from build123d import *

# Parameters (mm, degrees)
SKETCH1_W           = 55
SKETCH1_H           = 50
SKETCH1_R           = 6
SKETCH1_R_2         = 1.5
BOSS_EXTRUDE1_DEPTH = 5
SKETCH2_W           = 5.5
SKETCH2_H           = 2
SKETCH2_W_2         = 3
SKETCH2_H_2         = 12
CUT_EXTRUDE1_DEPTH  = 5
SKETCH3_W           = 5
SKETCH3_H           = 60
SKETCH3_W_2         = 26.5
SKETCH3_H_2         = 5
BOSS_EXTRUDE2_DEPTH = 5


with BuildPart() as part:
    # Sketch1 → Boss-Extrude1 (new body)
    with BuildSketch(Plane.XY):
        with Locations((0, -2)):
            Rectangle(SKETCH1_W, SKETCH1_H)
        with Locations((0, -7)):
            Circle(SKETCH1_R, mode=Mode.SUBTRACT)
        with Locations((-15.5, 0)):
            Circle(SKETCH1_R_2, mode=Mode.SUBTRACT)
        with Locations((-7.75, 13.423393759)):
            Circle(SKETCH1_R_2, mode=Mode.SUBTRACT)
        with Locations((7.75, 13.423393759)):
            Circle(SKETCH1_R_2, mode=Mode.SUBTRACT)
        with Locations((15.5, 0)):
            Circle(SKETCH1_R_2, mode=Mode.SUBTRACT)
        with Locations((7.75, -13.423393759)):
            Circle(SKETCH1_R_2, mode=Mode.SUBTRACT)
        with Locations((-7.75, -13.423393759)):
            Circle(SKETCH1_R_2, mode=Mode.SUBTRACT)
    extrude(amount=BOSS_EXTRUDE1_DEPTH)

    # Sketch2 → Cut-Extrude1 (cut)
    with BuildSketch(Plane.XY.offset(5)):
        with Locations((-19.75, -21)):
            Rectangle(SKETCH2_W, SKETCH2_H)
        with Locations((19.75, -21)):
            Rectangle(SKETCH2_W, SKETCH2_H)
        with Locations((-19.75, -21)):
            Rectangle(SKETCH2_W_2, SKETCH2_H_2)
        with Locations((19.75, -21)):
            Rectangle(SKETCH2_W_2, SKETCH2_H_2)
        with Locations((19.75, 17)):
            Rectangle(SKETCH2_W_2, SKETCH2_H_2)
        with Locations((-19.75, 17)):
            Rectangle(SKETCH2_W_2, SKETCH2_H_2)
        with Locations((19.75, 17)):
            Rectangle(SKETCH2_W, SKETCH2_H)
        with Locations((-19.75, 17)):
            Rectangle(SKETCH2_W, SKETCH2_H)
    extrude(amount=-CUT_EXTRUDE1_DEPTH, mode=Mode.SUBTRACT)

    # Sketch3 → Boss-Extrude2 (add)
    with BuildSketch(Plane.XY.offset(5)):
        with Locations((-28.75, -2)):
            Rectangle(SKETCH3_W, SKETCH3_H)
        with Locations((0, -29.5)):
            Rectangle(SKETCH3_W_2, SKETCH3_H_2)
        with Locations((28.75, -2)):
            Rectangle(SKETCH3_W, SKETCH3_H)
        with Locations((0, 25.5)):
            Rectangle(SKETCH3_W_2, SKETCH3_H_2)
    extrude(amount=-BOSS_EXTRUDE2_DEPTH)


solid = part.part
Input: part model. Units: mm. Frame: model coordinates. A direction names the side the tool comes from. Round coordinates to 2 decimals unless told otherwise and drop trailing zeros. Order: outer loops, then holes, each group sorted by start corner. A loop starts at its lowest first (then second) coordinate and runs counter-clockwise, first axis right, second up. Notation, with made-up numbers: (35, 74) - (53, 74) arc R30 ccw to (53, 113) - close; hole circle Ø6 at (27.5, 56.5). An arc over 180 degrees is marked (long way). Use a Markdown table: item, result.
1. Section D-D on y = 19. Return the cut outline in (x, z).
Evaluation:
| item | result |
|---|---|
| outline | (-31.25, 0) - (-21.25, 0) - (-21.25, 5) - (-31.25, 5) - close; (-18.25, 0) - (18.25, 0) - (18.25, 5) - (-18.25, 5) - close; (21.25, 0) - (31.25, 0) - (31.25, 5) - (21.25, 5) - close |
2. Material intervals for probe 1 along X at (y, z) = (-25, 3.65); probe 2 along Y at (x, z) = (7.75, 1.95); probe 3 along X at (y, z) = (-27.5, 1.35), sorted ascending.
Evaluation:
| item | result |
|---|---|
| probe 1 | -31.25 to -21.25, -18.25 to 18.25, 21.25 to 31.25 |
| probe 2 | -32 to -14.92, -11.92 to 11.92, 14.92 to 28 |
| probe 3 | -31.25 to -26.25, -13.25 to 13.25, 26.25 to 31.25 |
3. Section C-C on x = -7.75. Return the cut outline in (y, z).
Evaluation:
| item | result |
|---|---|
| outline | (-32, 0) - (-14.92, 0) - (-14.92, 5) - (-32, 5) - close; (-11.92, 0) - (11.92, 0) - (11.92, 5) - (-11.92, 5) - close; (14.92, 0) - (28, 0) - (28, 5) - (14.92, 5) - close |
4. Access query for faces 4 (the face through (21.25, 20, 3)), 5 (the face through (22.5, -21, 3)), 6 (the face through (-31.25, -2, 3)), 7 (the face through (-16, -27, 2)), 8 (the face through (31.25, -2, 3)). Directions: +Z, -Z, +X, -X, +Y, -Y. A direction counts if a zero-diameter tool reaches every point of the face in a straight line with its end or side. Return the directions, or none.
Evaluation:
| item | result |
|---|---|
| face 4 | +Z, -Z, +Y |
| face 5 | +Z, -Z |
| face 6 | +Z, -Z, -X, +Y, -Y |
| face 7 | +Z, -Z, -Y |
| face 8 | +Z, -Z, +X, +Y, -Y |
5. Section A-A on x = -15.5. Return the cut outline in (y, z), then the cut area to 3 significant figures.
Evaluation:
| item | result |
|---|---|
| outline | (-27, 0) - (-1.5, 0) - (-1.5, 5) - (-27, 5) - close; (1.5, 0) - (23, 0) - (23, 5) - (1.5, 5) - close |
| area | 235 mm^2 |
6. Section B-B on y = -7. Return the cut outline in (x, z), then the cut area to 4 significant figures.
Evaluation:
| item | result |
|---|---|
| outline | (-31.25, 0) - (-6, 0) - (-6, 5) - (-31.25, 5) - close; (6, 0) - (31.25, 0) - (31.25, 5) - (6, 5) - close |
| area | 252.5 mm^2 |
7. First-contact query: pin 1 (1 mm diameter, centred on x = 17.5, z = 3, fed in from +Y); pin 2 (2.5 mm diameter, centred on x = 23, z = 2, fed in from -Y). Flat tips, straight axial feed; report the tip coordinate or a pass-through.
Evaluation:
| item | result |
|---|---|
| pin 1 | y = 23 |
| pin 2 | y = -27 |
8. Mould query, pull axis Y, two halves, no side actions, for faces 1 (the face through (14, 0, 2)), 2 (the face through (-16, 23, 2)), 3 (the face through (-29, -32, 3)). Classes: +Y half, -Y half, draft (parallel to the pull), parting line (faces both ways), or undercut.
Evaluation:
| item | result |
|---|---|
| face 1 | undercut |
| face 2 | +Y half |
| face 3 | -Y half |
